from build123d import *

# Parameters (mm, degrees)
SKETCH014_R     = 3.5
SKETCH014_R_2   = 1.3
SKETCH014_W     = 14.1
SKETCH014_H     = 14.1
PAD004_DEPTH    = 3
SKETCH015_R     = 2.5
POCKET009_DEPTH = 1
SKETCH016_W     = 13
SKETCH016_H     = 15
POCKET010_DEPTH = 2


with BuildPart() as part:
    # Sketch014 → Pad004 (new body)
    with BuildSketch(Plane.XY):
        with BuildLine():
            Line((0, 0), (57, 0))
            Line((57, 0), (57, 95))
            Line((57, 95), (0, 95))
            Line((0, 73.306976), (0, 95))
            ThreePointArc((0, 73.306976), (-18, 47.5), (0, 21.693024))
            Line((0, 21.693024), (0, 0))
        make_face()
        with Locations((9.5, 47.5)):
            Circle(SKETCH014_R, mode=Mode.SUBTRACT)
        with Locations((19, 85.5)):
            Circle(SKETCH014_R_2, mode=Mode.SUBTRACT)
        with Locations((38, 85.5)):
            Circle(SKETCH014_R_2, mode=Mode.SUBTRACT)
        with Locations((38, 66.5)):
            Circle(SKETCH014_R_2, mode=Mode.SUBTRACT)
        with Locations((19, 66.5)):
            Circle(SKETCH014_R_2, mode=Mode.SUBTRACT)
        with Locations((38, 28.5)):
            Circle(SKETCH014_R_2, mode=Mode.SUBTRACT)
        with Locations((19, 28.5)):
            Circle(SKETCH014_R_2, mode=Mode.SUBTRACT)
        with Locations((19, 9.5)):
            Circle(SKETCH014_R_2, mode=Mode.SUBTRACT)
        with Locations((38, 9.5)):
            Circle(SKETCH014_R_2, mode=Mode.SUBTRACT)
        with Locations((47.5, 19)):
            Circle(SKETCH014_R_2, mode=Mode.SUBTRACT)
        with Locations((47.5, 76)):
            Circle(SKETCH014_R_2, mode=Mode.SUBTRACT)
        with Locations((9.5, 9.5)):
            Rectangle(SKETCH014_W, SKETCH014_H, mode=Mode.SUBTRACT)
        with Locations((28.5, 9.5)):
            Rectangle(SKETCH014_W, SKETCH014_H, mode=Mode.SUBTRACT)
        with Locations((47.5, 9.5)):
            Rectangle(SKETCH014_W, SKETCH014_H, mode=Mode.SUBTRACT)
        with Locations((47.5, 28.5)):
            Rectangle(SKETCH014_W, SKETCH014_H, mode=Mode.SUBTRACT)
        with Locations((47.5, 66.5)):
            Rectangle(SKETCH014_W, SKETCH014_H, mode=Mode.SUBTRACT)
        with Locations((47.5, 85.5)):
            Rectangle(SKETCH014_W, SKETCH014_H, mode=Mode.SUBTRACT)
        with Locations((28.5, 85.5)):
            Rectangle(SKETCH014_W, SKETCH014_H, mode=Mode.SUBTRACT)
        with Locations((9.5, 85.5)):
            Rectangle(SKETCH014_W, SKETCH014_H, mode=Mode.SUBTRACT)
    extrude(amount=PAD004_DEPTH)

    # Sketch015 (on Face51 of Pad004) → Pocket009 (cut)
    with BuildSketch(Plane.XY.offset(3)):
        with Locations((19, 28.5)):
            Circle(SKETCH015_R)
        with Locations((38, 28.5)):
            Circle(SKETCH015_R)
        with Locations((47.5, 19)):
            Circle(SKETCH015_R)
        with Locations((38, 9.5)):
            Circle(SKETCH015_R)
        with Locations((19, 9.5)):
            Circle(SKETCH015_R)
        with Locations((19, 66.5)):
            Circle(SKETCH015_R)
        with Locations((38, 85.5)):
            Circle(SKETCH015_R)
        with Locations((38, 66.5)):
            Circle(SKETCH015_R)
        with Locations((47.5, 76)):
            Circle(SKETCH015_R)
        with Locations((19, 85.5)):
            Circle(SKETCH015_R)
    extrude(amount=-POCKET009_DEPTH, mode=Mode.SUBTRACT)

    # Sketch016 (on Face4 of Pocket009) → Pocket010 (cut)
    with BuildSketch(Plane(origin=(0, 0, 0), x_dir=(1, 0, 0), z_dir=(0, 0, -1))):
        with Locations((9.5, -47.5)):
            Rectangle(SKETCH016_W, SKETCH016_H)
    extrude(amount=-POCKET010_DEPTH, mode=Mode.SUBTRACT)


with BuildPart() as part_1:
    # Body002 placement: moved
    add(part.part.moved(Location((6, 6, 11))))


solid = part_1.part
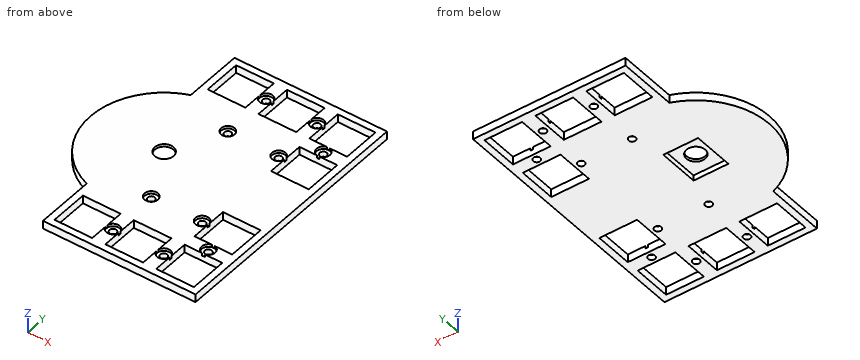
Source: CAD feature listing. Evaluate the final solid. Frame: model axes, mm. Coordinates: 2 decimals unless noted, no trailing zeros. Loops run counter-clockwise (first coordinate to the right, second up) from the corner with the lowest first, then second, coordinate; pieces in that order, holes last. Notation, with made-up numbers: (-6.5, 3) - (47.5, 3) arc R30 cw to (47.5, 29) - close; hole circle Ø8 at (57.5, 52.5). An arc over 180 degrees is marked (long way). One line per item, written item: value. Start each with the question number.
1. Section C-C (z = 12.35). State how many separate pieces and enclosed holes the cut face has, and give its area (3 significant figures).
2. Section B-B (x = 36). Return the cut outline in (y, z).
3. Section A-A (y = 25). Return the cut outline in (x, z).
4. Contact query for flat-ended pins moving along their axis: P1, Ø1.6, axis at x = 44, y = 72.5, coming from the +Z side; P2, Ø3.5, axis at x = 53.5, y = 25, coming from the +Z side. Output: stop coordinate, or through.
5. Ray query, L1, parallel to X at y = 86, z = 13.2; L2, parallel to X at y = 15.5, z = 11.8; L3, parallel to Y at x = 55, z = 12.3. Return the intervals inside material, ascending.
Verdict:
1. separate pieces: 1
1. enclosed holes: 19
1. area: 4,250 mm2
2. outline: (6, 11) - (8.45, 11) - (8.45, 14) - (6, 14) - close; (22.55, 11) - (84.45, 11) - (84.45, 14) - (22.55, 14) - close; (98.55, 11) - (101, 11) - (101, 14) - (98.55, 14) - close
3. outline: (6, 11) - (52.2, 11) - (52.2, 13) - (51, 13) - (51, 14) - (6, 14) - close; (54.8, 11) - (63, 11) - (63, 14) - (56, 14) - (56, 13) - (54.8, 13) - close
4. P1: passes through
4. P2: stops at z = 13
5. L1: x = 6 to 8.45, 22.55 to 27.45, 41.55 to 46.45, 60.55 to 63
5. L2: x = 6 to 8.45, 22.55 to 23.7, 26.3 to 27.45, 41.55 to 42.7, 45.3 to 46.45, 60.55 to 63
5. L3: y = 6 to 8.45, 22.55 to 27.45, 41.55 to 65.45, 79.55 to 84.45, 98.55 to 101
